For this review, take the finished solid that the model builds, in its own axes (mm). A direction names the side the tool comes from. Round coordinates to 2 decimals unless told otherwise and drop trailing zeros. Order: outer loops, then holes, each group sorted by start corner. A loop starts at its lowest first (then second) coordinate and runs counter-clockwise, first axis right, second up. Notation, with made-up numbers: (80, 60) - (94, 60) arc R22 ccw to (94, 84) - close; hole circle Ø2 at (86.5, -35). An arc over 180 degrees is marked (long way). Write each question's results on one line, items separated by ' | '. Start each with the question number.
(1) Take a section at C-C, the plane x = 7. Give the boundary of the cut face in (y, z), plus the area to 3 significant figures.
(2) For L1, parallel to Z at x = 15, y = 23.5; L2, parallel to Y at x = 14, z = 11; L3, parallel to X at y = -7, z = 30.5, list the stretches that pass through material, from the lowest coordinate up. Write a range as from..to.
(3) Insertion check: pin 1 Ø2 at (x, z) = (-5, 24.5) entering from -Y; pin 2 Ø1.5 at (x, z) = (-9, 29) entering from +Y; pin 3 Ø6 at (x, z) = (-12, 9.5) entering from -Y. Each pin has a flat end and moves straight along its axis. Give the tip position at first contact, or say it passes through.
(4) Take a section at A-A, the plane y = 0. Give the boundary of the cut face in (x, z).
(5) Take a section at D-D, the plane z = 16. Give the boundary of the cut face in (x, y).
(6) Take a section at B-B, the plane z = 24.5. Give the boundary of the cut face in (x, y), plus the area to 3 significant figures.
(7) For faces 1 (the flat face through (-7.65, -37.17, 9.81)), 2 (the flat face through (12, 0, 20)), 3 (the flat face through (1.674, -37.173, 12.622)), 4 (the flat face through (10.585, -37.173, 8.22)), 5 (the flat face through (1.261, -37.173, 5.413)), list the 3-axis set-ups (+Z, -Z, +X, -X, +Y, -Y) from which the entire face can be reached by the end or side of a thin tool; tool diameter is ignored.
Autodesk Fusion 360 part; units mm, degrees
sketch "Sketch1" plane through (0, 0, 0) normal (0, 0, 1) x (1, 0, 0)
  line L0 (27.6067, 32.2429) -> (-27.6067, 32.2429)
  line L1 (-27.6067, 32.2429) -> (-27.6067, -32.2429)
  line L2 (-27.6067, -32.2429) -> (27.6067, -32.2429)
  line L3 (27.6067, -32.2429) -> (27.6067, 32.2429)
  line L4 (27.6067, 32.2429) -> (-27.6067, -32.2429) construction
  line L5 (-27.6067, 32.2429) -> (27.6067, -32.2429) construction
extrude "Extrude1" add sketch "Sketch1" along normal blind 20
sketch "Sketch2" plane through (0, 0, 20) normal (0, 0, 1) x (-1, 0, 0)
  line L0 (-27.6067, 32.2429) -> (-27.6067, -32.2429)
  line L1 (-27.6067, -32.2429) -> (27.6067, -32.2429)
  line L2 (27.6067, -32.2429) -> (27.6067, 32.2429)
  line L3 (27.6067, 32.2429) -> (-27.6067, 32.2429)
  circle A0 centre (0, 0) radius 11.8335
extrude "Extrude2" add sketch "Sketch2" along normal blind 20 contours A0
sketch "Sketch4" plane through (0, -32.2429, 0) normal (0, -1, 0) x (1, 0, 0)
  line L0 (-27.6067, 0) -> (27.6067, 0)
  line L1 (27.6067, 0) -> (27.6067, 20)
  line L2 (27.6067, 20) -> (-27.6067, 20)
  line L3 (-27.6067, 20) -> (-27.6067, 0)
  line L4 (-7.3118, 13.4579) -> (10.9147, 11.7624)
  line L5 (10.9147, 11.7624) -> (10.2462, 4.5769)
  line L6 (10.2462, 4.5769) -> (-7.9802, 6.2724)
  line L7 (-7.9802, 6.2724) -> (-7.3118, 13.4579)
extrude "Extrude4" add sketch "Sketch4" along normal blind 10 contours L4 L5 L6 L7
sketch "Sketch3" plane through (0, 0, 40) normal (0, 0, 1) x (-1, 0, 0)
  circle A0 centre (0, 0) radius 11.8335
  circle A1 centre (0, 0) radius 4.7343
extrude "Extrude3" [suppressed]
Results below:
1) outline: (-42.24, 4.88) - (-32.24, 4.88) - (-32.24, 0) - (32.24, 0) - (32.24, 20) - (9.54, 20) - (9.54, 40) - (-9.54, 40) - (-9.54, 20) - (-32.24, 20) - (-32.24, 12.13) - (-42.24, 12.13) - close | area: 1,740 mm^2
2) L1: z = 0..20 | L2: y = -32.24..32.24 | L3: x = -9.54..9.54
3) pin 1: stops at y = -11.14 | pin 2: stops at y = 8.48 | pin 3: stops at y = -32.24
4) outline: (-27.61, 0) - (27.61, 0) - (27.61, 20) - (11.83, 20) - (11.83, 40) - (-11.83, 40) - (-11.83, 20) - (-27.61, 20) - close
5) outline: (-27.61, -32.24) - (27.61, -32.24) - (27.61, 32.24) - (-27.61, 32.24) - close
6) outline: circle Ø23.67 at (0, 0) | area: 440 mm^2
7) face 1: +Z, -X, -Y | face 2: +Z | face 3: +Z, +X, -Y | face 4: -Z, +X, -Y | face 5: -Z, -X, -Y
